Design review of the part built by this model. Coordinates are the model's own, in mm. Give positions to 0.01 mm unless a question says otherwise; leave off trailing zeros. Write each loop counter-clockwise with the first axis right and the second up, starting at its lowest first coordinate (ties: lowest second). Pieces come first, ordered by that corner, then holes. Notation, with made-up numbers: (-32.5, -39.5) - (-4.5, -39.5) arc R19 cw to (-4.5, -4.5) - close; hole circle Ø9 at (-33, 34.25). An arc over 180 degrees is marked (long way). Use a Markdown table: item, result. Add a question column.
```python
from build123d import *

# Parameters (mm, degrees)
SKETCH_1_W               = 150
SKETCH_1_H               = 150
EXTRUDE_1_DEPTH          = 6
FILLET_1_R               = 10
SKETCH_3_R               = 1.25
CUT_EXTRUDE_4_DEPTH      = 107.235587258
PATTERN_CIRCULAR_2_COUNT = 4
SKETCH_7_R               = 1.25
CUT_EXTRUDE_11_DEPTH     = 10
SKETCH_9_R               = 1.25
CUT_EXTRUDE_12_DEPTH     = 10
SKETCH_10_R              = 2.5
CUT_EXTRUDE_13_DEPTH     = 10


with BuildPart() as part:
    # 草图1 → 凸台-拉伸1 (new body)
    with BuildSketch(Plane(origin=(0, 0, 0), x_dir=(1, 0, 0), z_dir=(0, 1, 0))):
        Rectangle(SKETCH_1_W, SKETCH_1_H)
    extrude(amount=EXTRUDE_1_DEPTH)

    # 圆角1
    fillet_1_edges = [part.edges().sort_by_distance(p)[0] for p in [
        (75, 3, 75),
        (-75, 3, 75),
        (-75, 3, -75),
        (75, 3, -75),
    ]]
    fillet(fillet_1_edges, radius=FILLET_1_R)

    # 草图3 → 切除-拉伸4 (cut, through all)
    with BuildSketch(Plane.XZ):
        with Locations(Location((56.568542495, 56.568542495, 0), (0, 0, 270))):
            Circle(SKETCH_3_R)
    cut_extrude_4 = extrude(amount=-CUT_EXTRUDE_4_DEPTH, mode=Mode.SUBTRACT)

    # 阵列(圆周)2: 切除-拉伸4 ×4 about axis
    pattern_circular_2_axis = Axis((-0.01239132, 0, -0.01239132), (0, 1, 0))
    for i in range(1, PATTERN_CIRCULAR_2_COUNT):
        add(cut_extrude_4.rotate(pattern_circular_2_axis, i * 360 / PATTERN_CIRCULAR_2_COUNT), mode=Mode.SUBTRACT)

    # 草图7 → 切除-拉伸11 (cut)
    with BuildSketch(Plane.XZ):
        with Locations(Location((-36.593325134, -56.593325134, 0), (0, 0, 270))):
            Circle(SKETCH_7_R)
        with Locations(Location((36.568542495, -56.593325134, 0), (0, 0, 270))):
            Circle(SKETCH_7_R)
        with Locations(Location((-36.593325134, 56.568542495, 0), (0, 0, 270))):
            Circle(SKETCH_7_R)
        with Locations(Location((36.568542495, 56.568542495, 0), (0, 0, 270))):
            Circle(SKETCH_7_R)
    extrude(amount=-CUT_EXTRUDE_11_DEPTH, mode=Mode.SUBTRACT)

    # 草图9 → 切除-拉伸12 (cut)
    with BuildSketch(Plane.XZ):
        with Locations(Location((13.435028843, 13.435028843, 0), (0, 0, 270))):
            Circle(SKETCH_9_R)
        with Locations(Location((13.435028843, -13.435028843, 0), (0, 0, 270))):
            Circle(SKETCH_9_R)
        with Locations(Location((-13.435028843, -13.435028843, 0), (0, 0, 270))):
            Circle(SKETCH_9_R)
        with Locations(Location((-13.435028843, 13.435028843, 0), (0, 0, 270))):
            Circle(SKETCH_9_R)
    extrude(amount=-CUT_EXTRUDE_12_DEPTH, mode=Mode.SUBTRACT)

    # 草图10 → 切除-拉伸13 (cut)
    with BuildSketch(Plane.XZ):
        with Locations(Location((0, 0, 0), (0, 0, 270))):
            Circle(SKETCH_10_R)
    extrude(amount=-CUT_EXTRUDE_13_DEPTH, mode=Mode.SUBTRACT)


solid = part.part
```
(1) Add section B-B (x = 0). State the section outline as (y, z) points, and give its area (3 significant figures).
(2) For line 1 along X through (y, z) = (3.9, 0); line 2 along X through (y, z) = (5.5, -57.5); line 3 along X through (y, z) = (1.65, 2), list the stretches that pass through material, from the lowest coordinate up.
(3) Insertion check: pin 1 (2 mm diameter, centred on x = -13.44, z = -13.44, fed in from +Y). The pin has a flat end and moves straight along its axis. Give the tip position at first contact, or say it passes through.
(4) Mouldability with a two-part tool opening along Z and no side actions: class faces 1 (the face through (-72.15, 3.04, 71.99)), 2 (the face through (-1, 6, -18)), 3 (the face through (-2.44, 2.96, 0.54)), 4 (the face through (72.15, 3.04, -71.99)) as +Z half, -Z half, draft (parallel to the pull), parting line (faces both ways), or undercut.
(5) Add section A-A (z = 0). State the section outline as (x, y) points.
Answers follow:
| question | item | result |
|---|---|---|
| 1 | outline | (0, -75) - (6, -75) - (6, -2.5) - (0, -2.5) - close; (0, 2.5) - (6, 2.5) - (6, 75) - (0, 75) - close |
| 1 | area | 870 mm^2 |
| 2 | line 1 | -75 to -2.5, 2.5 to 75 |
| 2 | line 2 | -75 to -57.45, -55.73 to -37.45, -35.73 to 35.71, 37.43 to 55.71, 57.43 to 75 |
| 2 | line 3 | -75 to -1.5, 1.5 to 75 |
| 3 | pin 1 | through |
| 4 | face 1 | +Z half |
| 4 | face 2 | draft |
| 4 | face 3 | undercut |
| 4 | face 4 | -Z half |
| 5 | outline | (-75, 0) - (-2.5, 0) - (-2.5, 6) - (-75, 6) - close; (2.5, 0) - (75, 0) - (75, 6) - (2.5, 6) - close |
